Model file for the job. Use its own axes, mm. Face numbers are marked on the shaded views. Coordinates: 2 decimals unless noted, no trailing zeros. Order: outer loops, then holes, each group sorted by start corner. A loop starts at its lowest first (then second) coordinate and runs counter-clockwise, first axis right, second up. Notation, with made-up numbers: (64, 84.25) -> (79, 84.25) arc R25 ccw to (79, 119.25) -> close; hole circle Ø1 at (60, 28). An arc over 180 degrees is marked (long way). Write item = value, one per line. Start each with the question number.
Q1. Mould opens along Y. For the marked faces 1 and 2 say: +Y half, -Y half, draft (parallel to the pull), parting line (faces both ways), or undercut.
Q2. Flat gauge pins, fed straight in: pin 1 (3 mm diameter, centred on y = 0, z = 5, fed in from +X); pin 2 (4.5 mm diameter, centred on x = 17, z = 4, fed in from -Y); pin 3 (1.6 mm diameter, centred on y = -1.5, z = 4.5, fed in from -X); pin 4 (2.5 mm diameter, centred on x = 15.5, z = 6.5, fed in from -Y). Where does each tip first touch, or does it go through?
Q3. Wall check: line 1 (X direction, y = 22, z = 7); line 2 (Z direction, x = 3, y = 25). Give the ranges that are in metal, low to high. Write a range as from..to.
Q4. Cut at A-A, the plane x = 25.5. List the corners of the cut face in (y, z), plus the area to 3 significant figures.
Q5. Cut at B-B, the plane z = 5. List the corners of the cut face in (x, y).
from build123d import *

# Parameters (mm, degrees)
F0_W        = 120
F0_H        = 120
F1_DEPTH    = 3
F2_W        = 113
F2_H        = 113
F3_DEPTH    = 5
F4_T        = 2.5
F4_T3_DEPTH = 118
F4_T5_DEPTH = 118


# Not quite as in the source:
# - a shell that OpenCascade refuses in one call is made with other operations: the cavity is built on its own and cut out


with BuildPart() as f1:
    # F0 (on Top) → F1 (new body)
    with BuildSketch(Plane.XY):
        Rectangle(F0_W, F0_H)
    extrude(amount=F1_DEPTH)

    # F2 (on face) → F3 (join)
    with BuildSketch(Plane.XY.offset(3)):
        Rectangle(F2_W, F2_H)
    extrude(amount=F3_DEPTH)

    # F4: shell of thickness 2.5, made by hand


with BuildPart() as f4_core1:
    # F4_t2: copy of F1
    add(f1.part)

    # the walls: a layer under each face that stays
    f4_faces = [f4_core1.faces().sort_by_distance(p)[0] for p in [
        (0, -60, 1.5),
        (-60, 0, 1.5),
        (60, 0, 1.5),
        (0, 0, 0),
        (41.25, -58.5185185185, 3),
        (0, 60, 1.5),
        (0, -56.5, 5.5),
        (56.5, 0, 5.5),
        (0, 56.5, 5.5),
        (-56.5, 0, 5.5),
    ]]
    thicken(f4_faces, amount=-F4_T, mode=Mode.SUBTRACT)

    # F4_s4 → F4_t3 (cut)
    with BuildSketch(Plane.YZ.offset(-59)):
        Polygon((-56.525, 3.025), (-56.5, 0.5), (-54, 0.5), (-54, 3), align=None)
        Polygon((56.525, 3.025), (56.5, 0.5), (54, 0.5), (54, 3), align=None)
    extrude(amount=F4_T3_DEPTH, mode=Mode.SUBTRACT)

    # F4_s6 → F4_t5 (cut)
    with BuildSketch(Plane.XZ.offset(-59)):
        Polygon((56.525, 3.025), (56.5, 0.5), (54, 0.5), (54, 3), align=None)
        Polygon((-56.525, 3.025), (-56.5, 0.5), (-54, 0.5), (-54, 3), align=None)
    extrude(amount=F4_T5_DEPTH, mode=Mode.SUBTRACT)


with BuildPart() as f1_1:
    add(f1.part)

    # what is left inside the walls is the cavity
    f4_cavity = [f4_core1.part.solids().sort_by_distance(p)[0] for p in [
        (0, -18, 2.525),
    ]]
    add(f4_cavity, mode=Mode.SUBTRACT)


solid = f1_1.part
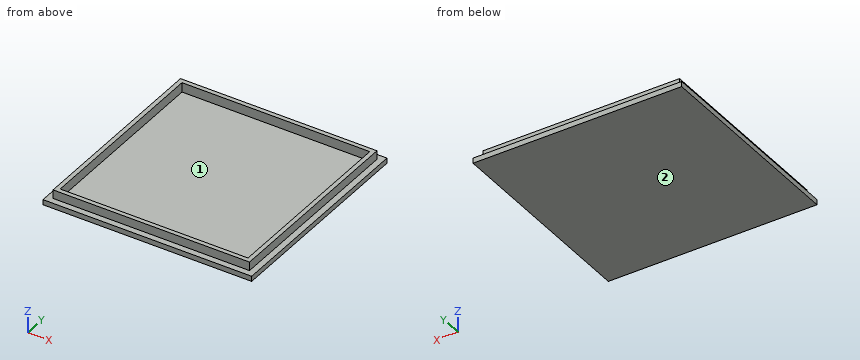
Here are the results:
q1.face_1 = undercut
q1.face_2 = draft
q2.pin_1 = 56.5
q2.pin_2 = -60
q2.pin_3 = -56.5
q2.pin_4 = -56.5
q3.line_1 = -56.5..-54, 54..56.5
q3.line_2 = 0..2.5
q4.outline = (-60, 0) -> (60, 0) -> (60, 3) -> (56.5, 3) -> (56.5, 8) -> (54, 8) -> (54, 2.5) -> (-54, 2.5) -> (-54, 8) -> (-56.5, 8) -> (-56.5, 3) -> (-60, 3) -> close
q4.area = 331 mm²
q5.outline = (-56.5, -56.5) -> (56.5, -56.5) -> (56.5, 56.5) -> (-56.5, 56.5) -> close; hole (-54, -54) -> (54, -54) -> (54, 54) -> (-54, 54) -> close
